Input: part model. Units: mm. Frame: model coordinates. Face numbers are marked on the shaded views. A direction names the side the tool comes from. Give positions to 0.01 mm unless a question says otherwise; leave off trailing zeros. Loops run counter-clockwise (first coordinate to the right, second up) from the corner with the lowest first, then second, coordinate; pieces in that order, holes last.
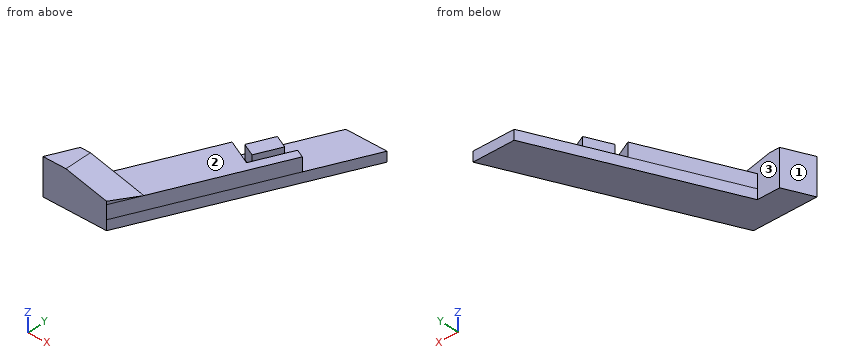
from build123d import *

# Parameters (mm, degrees)
BOSS_EXTRUDE1_DEPTH = 4
BOSS_EXTRUDE2_DEPTH = 5.5
BOSS_EXTRUDE3_DEPTH = 5.26
CUT_EXTRUDE1_DEPTH  = 25.26
SKETCH5_W           = 16.298124665
SKETCH5_H           = 32.903045357
BOSS_EXTRUDE4_DEPTH = 10
SKETCH6_W           = 73.83328153
SKETCH6_H           = 41.567802575
CUT_EXTRUDE2_DEPTH  = 120
SKETCH7_W           = 16.298124665
SKETCH7_H           = 10
CUT_EXTRUDE3_DEPTH  = 120


with BuildPart() as part:
    # Sketch1 → Boss-Extrude1 (new body)
    with BuildSketch(Plane.XY):
        Polygon((6.798067323, 45.385579117), (-26.566371189, -24.564420883), (-35.429799542, -24.564420883), (-40.556683823, -35.313157307), (-15.371402202, -35.313157307), (23.119920592, 45.385579117), align=None)
    boss_extrude1 = extrude(amount=-BOSS_EXTRUDE1_DEPTH)

    # Sketch2 → Boss-Extrude2 (add)
    with BuildSketch(Plane(origin=(0, 0, -4), x_dir=(-1, 0, 0), z_dir=(0, 0, -1))):
        Polygon((5.218881417, 14.259069333), (0.74156601, 23.645956291), (-4.312911582, 21.235094148), (0.164403825, 11.848207191), align=None)
        Polygon((40.556683823, -35.313157307), (35.429799542, -24.564420883), (26.566371189, -24.564420883), (8.815605583, 12.650833126), (-1.251818738, 7.848918048), (-8.260923666, 22.543811707), (-11.490263359, 21.003495686), (15.371402202, -35.313157307), align=None)
    boss_extrude2 = extrude(amount=BOSS_EXTRUDE2_DEPTH)

    # Sketch3 → Boss-Extrude3 (add)
    with BuildSketch(Plane(origin=(0, 0, -9.5), x_dir=(-1, 0, 0), z_dir=(0, 0, -1))):
        Polygon((40.556683823, -35.313157307), (35.429799542, -24.564420883), (10.244517921, -24.564420883), (15.371402202, -35.313157307), align=None)
    boss_extrude3 = extrude(amount=BOSS_EXTRUDE3_DEPTH)

    # Sketch4 → Cut-Extrude1 (cut)
    with BuildSketch(Plane.XZ.offset(35.313157307)):
        Polygon((-31.448639935, -14.76), (-10.244517921, -9.5), (-10.244517921, -14.76), align=None)
    cut_extrude1 = extrude(amount=-CUT_EXTRUDE1_DEPTH, mode=Mode.SUBTRACT)


with BuildPart() as body_2:
    # Sketch5 → Boss-Extrude4 (new body)
    with BuildSketch(Plane(origin=(0, 45.385579117, 0), x_dir=(1, 0, 0), z_dir=(0, 1, 0))):
        with Locations((14.947129656, -12.451522679)):
            Rectangle(SKETCH5_W, SKETCH5_H)
    extrude(amount=BOSS_EXTRUDE4_DEPTH)

    # Mirror8: Boss-Extrude1, Boss-Extrude2, Boss-Extrude3, Cut-Extrude1 across plane
    add(boss_extrude1.mirror(Plane.XY.offset(12.451522678)))
    add(boss_extrude2.mirror(Plane.XY.offset(12.451522678)))
    add(boss_extrude3.mirror(Plane.XY.offset(12.451522678)))
    add(cut_extrude1.mirror(Plane.XY.offset(12.451522678)), mode=Mode.SUBTRACT)


with BuildPart() as cut_extrude2_tool:
    # Sketch6 → Cut-Extrude2 (new body)
    with BuildSketch(Plane.XZ.offset(35.313157307)):
        with Locations((-3.640043058, 4.119144069)):
            Rectangle(SKETCH6_W, SKETCH6_H)
    extrude(amount=-CUT_EXTRUDE2_DEPTH)


with BuildPart() as part_1:
    add(part.part)

    # Cut-Extrude2: cut by cut_extrude2_tool
    add(cut_extrude2_tool.part, mode=Mode.SUBTRACT)


with BuildPart() as body_2_1:
    add(body_2.part)

    # Cut-Extrude2: cut by cut_extrude2_tool
    add(cut_extrude2_tool.part, mode=Mode.SUBTRACT)

    # Sketch7 → Cut-Extrude3 (cut)
    with BuildSketch(Plane.XY.offset(28.903045357)):
        with Locations((14.947129656, 50.385579117)):
            Rectangle(SKETCH7_W, SKETCH7_H)
    extrude(amount=-CUT_EXTRUDE3_DEPTH, mode=Mode.SUBTRACT)


solid = body_2_1.part
(1) Cut plane B-B (x = -19). Return the cut outline in (y, z), and give its area (3 significant figures).
Values follow:
outline: (-35.31, 24.9) - (-8.7, 24.9) - (-8.7, 34.4) - (-24.56, 34.4) - (-24.56, 36.57) - (-35.31, 36.57) - close
area: 276 mm2
(2) Cut plane C-C (y = 17.5). Return the cut outline in (x, z).
Values follow:
outline: (-6.5, 24.9) - (9.82, 24.9) - (9.82, 34.4) - (5.86, 34.4) - (5.86, 28.9) - (2.53, 28.9) - (2.53, 34.4) - (-3.67, 34.4) - (-3.67, 28.9) - (-6.5, 28.9) - close
(3) Pin query (flat end, axial travel): pin 1 Ø8 at (y, z) = (33, 32.5) entering from +X; pin 2 Ø2 at (y, z) = (33, 31.5) entering from +X; pin 3 Ø8 at (x, y) = (-4, 23.5) entering from +Z; pin 4 Ø3 at (x, z) = (-30.5, 28) entering from +Y. Return the tip coordinate at first contact, or that it passes through.
Values follow:
pin 1: stops at x = 18.05
pin 2: passes through
pin 3: stops at z = 34.4
pin 4: stops at y = -24.56
(4) Ray query, probe 1 along Z at (x, y) = (-17, -5); probe 2 along X at (y, z) = (8.5, 32.5); probe 3 along X at (y, z) = (20, 33.5). Return the intervals inside material, ascending.
Values follow:
probe 1: z = 24.9 to 34.4
probe 2: x = -10.8 to -0.11, 1.56 to 5.53
probe 3: x = -2.48 to 3.72, 7.05 to 11.01
(5) Cut plane A-A (z = 33). Return the cut outline in (x, y).
Values follow:
outline: (-40.56, -35.31) - (-15.37, -35.31) - (11.49, 21) - (8.26, 22.54) - (1.25, 7.85) - (-8.82, 12.65) - (-26.57, -24.56) - (-35.43, -24.56) - close; (-5.22, 14.26) - (-0.16, 11.85) - (4.31, 21.24) - (-0.74, 23.65) - close
(6) Cut plane D-D (z = 26.25). Return the cut outline in (x, y).
Values follow:
outline: (-40.56, -35.31) - (-15.37, -35.31) - (23.12, 45.39) - (6.8, 45.39) - (-26.57, -24.56) - (-35.43, -24.56) - close
(7) Reachability of the marked faces 1, 2 and 3 from +Z, -Z, +X, -X, +Y, -Y: full face, straight path, thin tool, end or side. Return the list, or none.
Values follow:
face 1: +Z, -Z, -X, +Y
face 2: +Z, +X, -X, +Y
face 3: +Z, -X, +Y
